from build123d import *

# Parameters (mm, degrees)
F1_DEPTH = 44.45
F2_W     = 63.5
F2_H     = 50.8
F3_DEPTH = 50.8


with BuildPart() as f1:
    # F0 (on Front) → F1 (new body, symmetric)
    with BuildSketch(Plane.XZ):
        with BuildLine():
            Line((-50.8, 12.7), (-50.8, -12.7))
            Line((-50.8, -12.7), (50.8, -12.7))
            Line((50.8, -12.7), (50.8, 12.7))
            ThreePointArc((50.8, 12.7), (0, 63.5), (-50.8, 12.7))
        make_face()
    extrude(amount=F1_DEPTH, both=True)

    # F2 (on Right) → F3 (cut, symmetric)
    with BuildSketch(Plane.YZ):
        with Locations((-0.797947, 38.1)):
            Rectangle(F2_W, F2_H)
    extrude(amount=F3_DEPTH, both=True, mode=Mode.SUBTRACT)


solid = f1.part
Build history of the part. All positions in model axes, mm. A direction names the side the tool comes from. Coordinates: 2 decimals unless noted, no trailing zeros. Order: outer loops, then holes, each group sorted by start corner. A loop starts at its lowest first (then second) coordinate and runs counter-clockwise, first axis right, second up. Notation, with made-up numbers: (-38.5, 66.25) -> (3.5, 66.25) arc R24 cw to (3.5, 100.25) -> close; hole circle Ø3 at (82.25, 18.25). An arc over 180 degrees is marked (long way). One line per item, written item: value.
(1) Probe line 1 (Y direction, x = 42.5, z = 36.5); line 2 (Z direction, x = 24, y = 20); line 3 (Z direction, x = 29.5, y = 40). List the from-to ranges inside material, lowest first. Write a range as [from, to].
Checked values:
line 1: [-44.45, -32.55], [30.95, 44.45]
line 2: [-12.7, 12.7]
line 3: [-12.7, 54.06]
(2) Mould opens along Y. For faces 1 (the flat face through (-1, -1, -12.7)), 2 (the flat face through (-1, 44.45, 17)), 3 (the flat face through (1, 30.952, 32)), 4 (the flat face through (1, -1, 12.7)) say: pulls with the +Y half, pulls with the -Y half, needs draft (parallel to the pull), parting line crosses it, or undercut.
Checked values:
face 1: needs draft
face 2: pulls with the +Y half
face 3: undercut
face 4: undercut
(3) Tool access for faces 5 (the cylindrical face through (1.117, -38.582, 63.488)), 6 (the flat face through (1, -32.548, 32)): list every direction of +Z, -Z, +X, -X, +Y, -Y with a clear straight run to the whole face (end or side of a thin tool).
Checked values:
face 5: +Z, +Y, -Y
face 6: +Z, +X, -X
(4) Slice it at D-D, the plane y = -19. List the corners of the cut face in (x, z), plus the area to 3 significant figures.
Checked values:
outline: (-50.8, -12.7) -> (50.8, -12.7) -> (50.8, 12.7) -> (-50.8, 12.7) -> close
area: 2,580 mm2
(5) Slice it at B-B, the plane x = 0. List the corners of the cut face in (y, z).
Checked values:
outline: (-44.45, -12.7) -> (44.45, -12.7) -> (44.45, 63.5) -> (30.95, 63.5) -> (30.95, 12.7) -> (-32.55, 12.7) -> (-32.55, 63.5) -> (-44.45, 63.5) -> close
(6) Slice it at A-A, the plane z = 17. List the corners of the cut face in (x, y), plus the area to 3 significant figures.
Checked values:
outline: (-50.62, -44.45) -> (50.62, -44.45) -> (50.62, -32.55) -> (-50.62, -32.55) -> close; (-50.62, 30.95) -> (50.62, 30.95) -> (50.62, 44.45) -> (-50.62, 44.45) -> close
area: 2,570 mm2
(7) Drop flat-ended pins along their axis: pin 1 Ø1.5 at (x, y) = (-19.5, 33) entering from +Z; pin 2 Ø12 at (x, y) = (31.5, -5.5) entering from +Z. Give the stop position or say it passes through.
Checked values:
pin 1: z = 59.91
pin 2: z = 12.7
(8) Slice it at C-C, the plane z = 27. List the corners of the cut face in (x, y).
Checked values:
outline: (-48.75, -44.45) -> (48.75, -44.45) -> (48.75, -32.55) -> (-48.75, -32.55) -> close; (-48.75, 30.95) -> (48.75, 30.95) -> (48.75, 44.45) -> (-48.75, 44.45) -> close
